Check sheet for the modelled part. Datum: model origin and axes. Units: mm. Round coordinates to 2 decimals unless told otherwise and drop trailing zeros. Write each loop counter-clockwise with the first axis right and the second up, starting at its lowest first coordinate (ties: lowest second). Pieces come first, ordered by that corner, then holes.
Autodesk Inventor part; units mm, degrees
ref_plane "YZ Plane" through (0, 0, 0) normal (1, 0, 0) x (0, 1, 0)
ref_plane "XZ Plane" through (0, 0, 0) normal (0, 1, 0) x (-1, 0, 0)
ref_plane "XY Plane" through (0, 0, 0) normal (0, 0, 1) x (1, 0, 0)
sketch "Sketch1" plane through (0, 0, 0) normal (0, 0, 1) x (1, 0, 0)
  line L0 (0, 0) -> (0, 6.35)
  line L1 (0, 6.35) -> (13.6118, 57.15)
  line L2 (13.6118, 57.15) -> (50.8, 47.1855)
  line L3 (50.8, 47.1855) -> (50.8, 0)
  line L4 (50.8, 0) -> (0, 0)
  dimension "d0" = 50.8
  dimension "d1" = 6.35
  dimension "d2" = 15
  dimension "d3" = 57.15
extrude "Extrusion1" add sketch "Sketch1" along normal mid plane 3.048
properties part number "A1-18002-100-54 Tube stop" material "Steel, Mild"
1. Sectioned sample at C-C, the plane y = 24.5. Enter the section's corners in (x, z), plus the area to 3 significant figures.
2. Scan lines: line 1 along X through (y, z) = (10.5, 1.25); line 2 along X through (y, z) = (37.5, 0.5); line 3 along Y through (x, z) = (47, 0.95). Record each from-to range of solid material in increasing order.
3. Sectioned sample at A-A, the plane z = 0.2. Enter the section's corners in (x, y).
4. Sectioned sample at B-B, the plane x = 31. Enter the section's corners in (y, z).
Computed values:
1. outline: (4.86, -1.52) - (50.8, -1.52) - (50.8, 1.52) - (4.86, 1.52) - close
1. area: 140 mm2
2. line 1: x = 1.11 to 50.8
2. line 2: x = 8.35 to 50.8
2. line 3: y = 0 to 48.2
3. outline: (0, 0) - (50.8, 0) - (50.8, 47.19) - (13.61, 57.15) - (0, 6.35) - close
4. outline: (0, -1.52) - (52.49, -1.52) - (52.49, 1.52) - (0, 1.52) - close
